Design review of the part built by this model. Coordinates are the model's own, in mm. Face numbers are marked on the shaded views. Round coordinates to 2 decimals unless told otherwise and drop trailing zeros. Order: outer loops, then holes, each group sorted by start corner. A loop starts at its lowest first (then second) coordinate and runs counter-clockwise, first axis right, second up. Notation, with made-up numbers: (23, 89) - (74, 89) arc R9 ccw to (74, 97) - close; hole circle Ø2 at (-38, 25). An arc over 180 degrees is marked (long way). Write item = value, one per line.
Autodesk Inventor part; units mm, degrees
ref_plane "YZ Plane" through (0, 0, 0) normal (1, 0, 0) x (0, 1, 0)
ref_plane "XZ Plane" through (0, 0, 0) normal (0, 1, 0) x (-1, 0, 0)
ref_plane "XY Plane" through (0, 0, 0) normal (0, 0, 1) x (1, 0, 0)
sketch "Sketch1" plane through (0, 0, 0) normal (0, 1, 0) x (-1, 0, 0)
  line L0 (-43, 27.5) -> (43, 27.5)
  line L1 (43, 27.5) -> (43, -27.5)
  line L2 (43, -27.5) -> (-43, -27.5)
  line L3 (-43, -27.5) -> (-43, 27.5)
  line L4 (-43, 27.5) -> (43, -27.5) construction
  line L5 (43, 27.5) -> (-43, -27.5) construction
  line L6 (43, -27.5) -> (46, -27.5)
  line L7 (46, -27.5) -> (46, 27.5)
  line L8 (46, 27.5) -> (43, 27.5)
  line L9 (43, 27.5) -> (43, -27.5)
  line L10 (-43, -27.5) -> (-46, -27.5)
  line L11 (-46, -27.5) -> (-46, 27.5)
  line L12 (-46, 27.5) -> (-43, 27.5)
  line L13 (-43, 27.5) -> (-43, -27.5)
  point P0 (0, 0)
  dimension "d0" = 86
  dimension "d1" = 55
  dimension "d2" = 3
  dimension "d3" = 55
  dimension "d4" = 3
extrude "Extrusion1" add sketch "Sketch1" along normal blind 3 contours L0 L1 L2 L3
extrude "Extrusion2" add sketch "Sketch1" along normal blind 3 contours L3 L10 L11 L12 | L8 L7 L6 L1
extrude "Extrusion3" add sketch "Sketch1" against normal blind 35 contours L3 L10 L11 L12 | L8 L7 L6 L1
sketch "Sketch2" plane through (46, 3, 27.5) normal (1, 0, 0) x (0, 0, -1)
  line L0 (0, -3) -> (0, -38)
  line L1 (0, -38) -> (55, -38)
  arc A0 (0, -38) -> (55, -38) centre (27.5, -28.794) ccw
  point P0 (27.5, -3)
  dimension "d11" = 29
extrude "Extrusion4" add sketch "Sketch2" against normal up to surface (3 mm away)
mirror "Mirror1" about plane through (0, 0, 0) normal (1, 0, 0) of "Extrusion4"
sketch "Sketch3" plane through (-46, 3, -27.5) normal (-1, 0, 0) x (0, 0, 1)
  circle A0 centre (27.5, -38) radius 4.5
  point P0 (27.5, -3)
  point P1 (0, -38)
  dimension "d14" = 9
extrude "Extrusion5" cut sketch "Sketch3" against normal blind 106.25
sketch "Sketch4" plane through (0, 3, 0) normal (0, 1, 0) x (1, 0, 0)
  line L0 (300, -250) -> (-300, -250)
  line L1 (-300, -250) -> (-300, 250)
  line L2 (-300, 250) -> (300, 250)
  line L3 (300, 250) -> (300, -250)
  line L4 (300, -250) -> (-300, 250) construction
  line L5 (-300, -250) -> (300, 250) construction
  line L6 (75, -65) -> (-75, -65)
  line L7 (-75, -65) -> (-75, 65)
  line L8 (-75, 65) -> (75, 65)
  line L9 (75, 65) -> (75, -65)
  line L10 (75, -65) -> (-75, 65) construction
  line L11 (-75, -65) -> (75, 65) construction
  line L12 (0, 250) -> (-40, 250)
  line L13 (-40, 250) -> (-40, 65)
  line L14 (0, 250) -> (40, 250)
  line L15 (40, 250) -> (40, 65)
  line L16 (300, 0) -> (300, 40)
  line L17 (300, 40) -> (75, 40)
  line L18 (300, 0) -> (300, -40)
  line L19 (300, -40) -> (75, -40)
  line L20 (0, -250) -> (-40, -250)
  line L21 (-40, -250) -> (-40, -65)
  line L22 (0, -250) -> (40, -250)
  line L23 (40, -250) -> (40, -65)
  line L24 (-300, 0) -> (-300, -40)
  line L25 (-300, -40) -> (-75, -40)
  line L26 (-300, 0) -> (-300, 40)
  line L27 (-300, 40) -> (-75, 40)
  line L28 (300, 40) -> (320, 40)
  line L29 (320, 40) -> (320, -40)
  line L30 (320, -40) -> (300, -40)
  line L31 (-300, 40) -> (-320, 40)
  line L32 (-320, 40) -> (-320, -40)
  line L33 (-320, -40) -> (-300, -40)
  line L34 (-40, 250) -> (-40, 270)
  line L35 (-40, 270) -> (40, 270)
  line L36 (40, 270) -> (40, 250)
  line L37 (-40, -250) -> (-40, -270)
  line L38 (-40, -270) -> (40, -270)
  line L39 (40, -270) -> (40, -250)
  point P0 (0, 0)
  dimension "d17" = 600
  dimension "d18" = 500
  dimension "d19" = 150
  dimension "d20" = 130
  dimension "d21" = 40
  dimension "d22" = 40
  dimension "d23" = 40
  dimension "d24" = 40
  dimension "d25" = 40
  dimension "d26" = 40
  dimension "d27" = 40
  dimension "d28" = 20
  dimension "d29" = 20
  dimension "d30" = 20
  dimension "d31" = 20
extrude "Extrusion6" add sketch "Sketch4" along normal blind 5 contours L0 L21 L6 L23 | L19 L9 L17 L3 | L6 L7 L8 L9 | L1 L27 L7 L25 | L15 L8 L13 L2
extrude "Extrusion7" add sketch "Sketch4" along normal blind 28 contours L39 L38 L37 L0 | L3 L28 L29 L30 | L33 L32 L31 L1 | L2 L34 L35 L36
fillet "Fillet1" radius 2 53 edges at (-40, 8, -157.5) (-40, 19.5, -250) (40, 19.5, -250) (40, 8, -157.5) (-57.5, 8, -65) (-75, 8, -52.5) (-187.5, 8, -40) (-300, 19.5, -40) (-300, 19.5, 40) (-187.5, 8, 40) (-75, 8, 52.5) (-57.5, 8, 65) (-40, 8, 157.5) (187.5, 8, -40) (75, 8, -52.5) (57.5, 8, -65) (40, 8, 157.5) (57.5, 8, 65) (75, 8, 52.5) (187.5, 8, 40) (300, 19.5, 40) (300, 19.5, -40) (-40, 19.5, 250) (40, 19.5, 250) (-300, 31, 0) (0, 31, -250) (300, 31, 0) (0, 31, 250) (0, 31, 270) (-40, 31, 260) (-310, 31, 40) (-310, 31, -40) (40, 31, 260) (310, 31, 40) (310, 31, -40) (320, 31, 0) (-40, 31, -260) (40, 31, -260) (0, 31, -270) (-320, 31, 0) (-320, 17, 40) (-40, 17, -270) (40, 17, -270) (-320, 17, -40) (320, 17, -40) (320, 17, 40) (-40, 17, 270) (40, 17, 270) (0, 3, 270) (300, 8, 0) (0, 8, 250) (0, 8, -250) (-300, 8, 0)
properties part number "atassolar" material "Aluminum 6061"
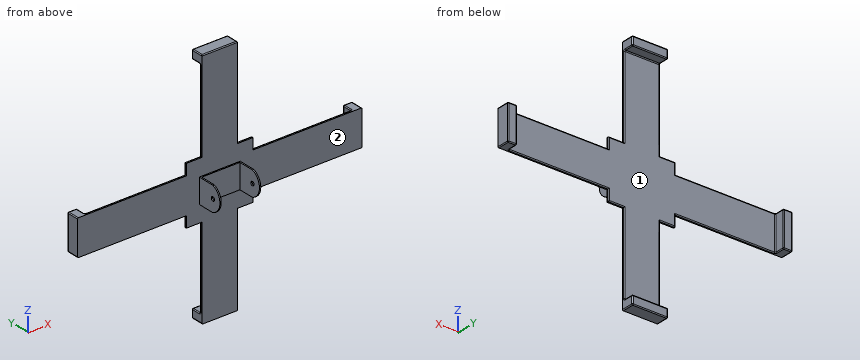
1) The part is to be moulded in two halves that separate along X. For the marked faces 1 and 2, say which applies: released by +X, released by -X, zero draft, split by the parting line, or undercut.
Findings:
face_1 = undercut
face_2 = zero draft
2) To check wall thickness, follow L1, parallel to Y at x = 44.45, z = 0; L2, parallel to X at y = 17, z = -30; L3, parallel to X at y = -13, z = -3.5. State the ranges of each line that lie inside material, in increasing order. Write a range as from..to.
Findings:
L1 = -54.79..-39.5, -30.5..8
L2 = -320..-300, 300..320
L3 = -46..-43, 43..46
3) We need section B-B on x = 164. Write out the cut boundary in (y, z).
Findings:
outline = (3, -40) - (6, -40) arc R2 ccw to (8, -38) - (8, 38) arc R2 ccw to (6, 40) - (3, 40) - close
4) We need section A-A on y = -23. Write out the cut boundary in (x, z).
Findings:
outline = (-46, -27.5) - (-43, -27.5) - (-43, 27.5) - (-46, 27.5) - close; (43, -27.5) - (46, -27.5) - (46, 27.5) - (43, 27.5) - close
5) Clearance check with flat-ended pins moving along their axes: pin 1 Ø8 at (x, y) = (251.5, 11.5) entering from +Z; pin 2 Ø1 at (x, y) = (-111, 5.5) entering from +Z; pin 3 Ø0.9 at (x, y) = (55, 4) entering from -Z. State where each tip first meets the part, or that it passes through.
Findings:
pin_1 = 39.32
pin_2 = 40
pin_3 = -65
6) We need section C-C on z = -205. Write out the cut boundary in (x, y), and give its area (3 significant figures).
Findings:
outline = (-40, 3) - (40, 3) - (40, 6) arc R2 ccw to (38, 8) - (-38, 8) arc R2 ccw to (-40, 6) - close
area = 398 mm^2
